Design review of the part shown in the three views and the two pictorial views. Dimensions are in mm from the part's minimum x, y and z. A direction names the side the tool comes from. Coordinates: 2 decimals unless noted, no trailing zeros. Loops run counter-clockwise (first coordinate to the right, second up) from the corner with the lowest first, then second, coordinate; pieces in that order, holes last. Notation, with made-up numbers: M 0.5,-25.75 L 59.5,-25.75 A12 ccw 59.5,-21.75 Z; hole C 37.25,78.25 d5. An arc over 180 degrees is marked long. Use one line per item in the form item = value.
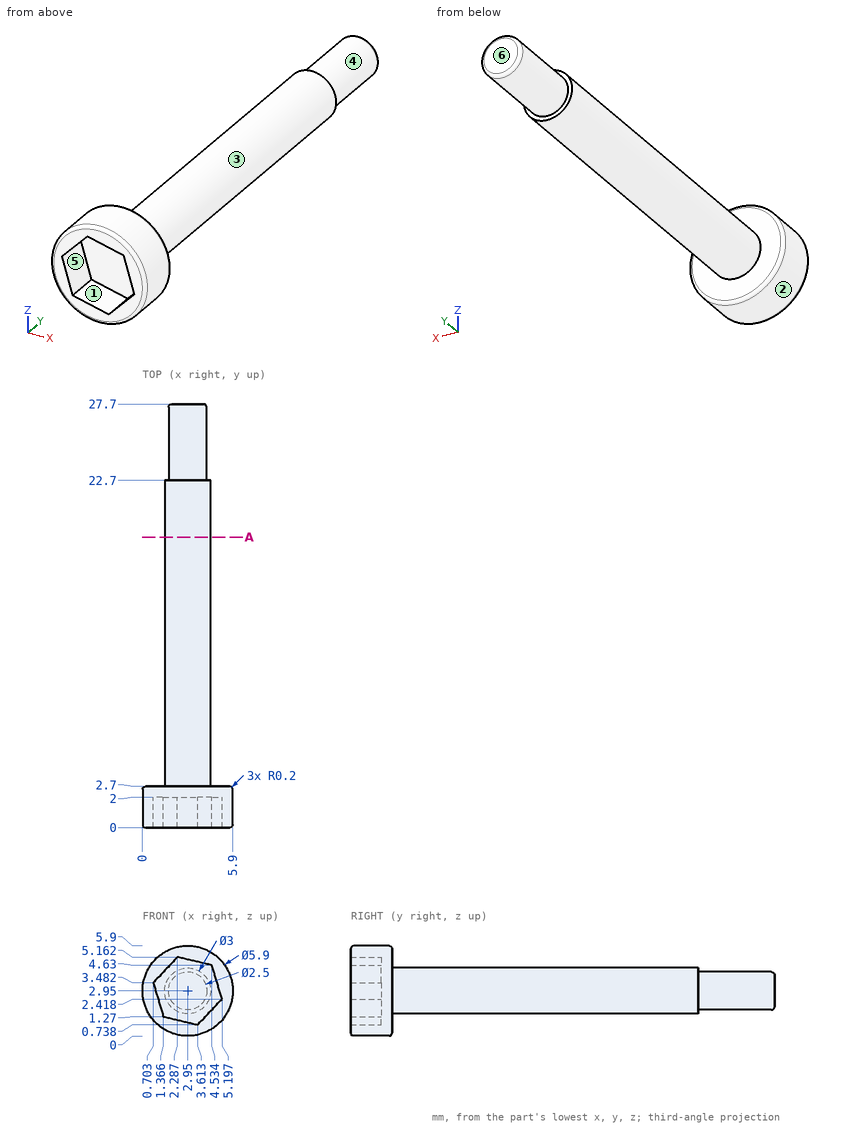
1. The part is to be moulded in two halves that separate along Z. For the marked faces 4, 5 and 6, say which applies: pulls with the +Z half, pulls with the -Z half, needs draft (parallel to the pull), parting line crosses it, or undercut.
Response values:
face_4 = parting line crosses it
face_5 = undercut
face_6 = needs draft
2. Add section A-A (y = 19). State the section outline as (x, z) points.
Response values:
outline = C 2.95,2.95 d3
3. Wall thickness on line 1 along Y through (x, z) = (3.75, 1.25); line 2 along Y through (x, z) = (3.3, 5.4); line 3 along Z through (x, y) = (3, 18): over which ranges is each line inside the solid? List them lowest first. Write a range as from..to.
Response values:
line_1 = 2..2.7
line_2 = 0..2.7
line_3 = 1.45..4.45
4. Machinability: for the marked faces 1, 2 and 3, which of the approach directions +Z, -Z, +X, -X, +Y, -Y give a long, thin tool a straight path to every point of the face, cutting with its end or side? Answer none if there is none.
Response values:
face_1 = -Y
face_2 = +Y, -Y
face_3 = +Y
